CAD build for the part. Positions are in the model's coordinates, mm. Round coordinates to 2 decimals unless told otherwise and drop trailing zeros. Write each loop counter-clockwise with the first axis right and the second up, starting at its lowest first coordinate (ties: lowest second). Pieces come first, ordered by that corner, then holes. Notation, with made-up numbers: M 21,-39.5 L 62,-39.5 A36 ccw 62,-4.5 Z; hole C 14,-15 d3. An arc over 180 degrees is marked long. Write each question's results on one line, items separated by ' | '. Start each with the question number.
```python
from build123d import *

# Parameters (mm, degrees)
SKETCH_1_R      = 22
SKETCH_1_R_2    = 17.5
EXTRUDE_1_DEPTH = 5
FILLET_1_R      = 0.25


with BuildPart() as part:
    # 草图1 → 凸台-拉伸1 (new body)
    with BuildSketch(Plane(origin=(0, 0, 0), x_dir=(1, 0, 0), z_dir=(0, 1, 0))):
        with Locations(Location((0, 0, 0), (0, 0, 270))):
            Circle(SKETCH_1_R)
        with Locations(Location((0, 0, 0), (0, 0, 270))):
            Circle(SKETCH_1_R_2, mode=Mode.SUBTRACT)
    extrude(amount=EXTRUDE_1_DEPTH)

    # 圆角1
    fillet_1_edges = [part.edges().sort_by_distance(p)[0] for p in [
        (0, 0, -22),
        (0, 5, -22),
        (0, 0, -17.5),
        (0, 5, -17.5),
    ]]
    fillet(fillet_1_edges, radius=FILLET_1_R)


solid = part.part
```
1) Saw through at A-A, the plane z = 0. Write the cut outline in (x, y), plus the area to 3 significant figures.
2) Saw through at B-B, the plane x = 0. Write the cut outline in (y, z).
3) Wall check: line 1 along X through (y, z) = (2.2, 0); line 2 along Z through (x, y) = (7, 2.1); line 3 along Z through (x, y) = (1.5, 4.35). Give the ranges that are in metal, low to high. Write a range as from..to.
4) Pull direction Z, two halves, no side cores. Call faces 1 (the face through (0, 0, -18)), 2 (the face through (-10.648, 2.468, -13.887)), 3 (the face through (-21.477, 2.468, -4.769)): pulls with the +Z half, pulls with the -Z half, needs draft (parallel to the pull), parting line crosses it, or undercut.
5) Saw through at C-C, the plane y = 2.65. Write the cut outline in (x, z).
6) Drop flat-ended pins along their axis: pin 1 Ø3 at (x, y) = (5.5, 1.5) entering from -Z; pin 2 Ø3 at (x, y) = (-13.5, 1) entering from +Z. Give the stop position or say it passes through.
Filled sheet:
1) outline: M -22,0.25 A0.25 ccw -21.75,0 L -17.75,0 A0.25 ccw -17.5,0.25 L -17.5,4.75 A0.25 ccw -17.75,5 L -21.75,5 A0.25 ccw -22,4.75 Z; M 17.5,0.25 A0.25 ccw 17.75,0 L 21.75,0 A0.25 ccw 22,0.25 L 22,4.75 A0.25 ccw 21.75,5 L 17.75,5 A0.25 ccw 17.5,4.75 Z | area: 44.9 mm^2
2) outline: M 0,-21.75 A0.25 ccw 0.25,-22 L 4.75,-22 A0.25 ccw 5,-21.75 L 5,-17.75 A0.25 ccw 4.75,-17.5 L 0.25,-17.5 A0.25 ccw 0,-17.75 Z; M 0,17.75 A0.25 ccw 0.25,17.5 L 4.75,17.5 A0.25 ccw 5,17.75 L 5,21.75 A0.25 ccw 4.75,22 L 0.25,22 A0.25 ccw 0,21.75 Z
3) line 1: x = -22..-17.5, 17.5..22 | line 2: z = -20.86..-16.04, 16.04..20.86 | line 3: z = -21.95..-17.44, 17.44..21.95
4) face 1: needs draft | face 2: undercut | face 3: parting line crosses it
5) outline: C 0,0 d44; hole C 0,0 d35
6) pin 1: stops at z = -21.63 | pin 2: stops at z = 18.44
